Design review of the part built by this model. Coordinates are the model's own, in mm. A direction names the side the tool comes from. Coordinates: 2 decimals unless noted, no trailing zeros. Write each loop counter-clockwise with the first axis right and the second up, starting at its lowest first coordinate (ties: lowest second). Pieces come first, ordered by that corner, then holes.
Q1. Add section B-B, the plane x = 21. Give the boundary of the cut face in (y, z).
Q2. Clearance check with flat-ended pins moving along their axes: pin 1 Ø8 at (y, z) = (4.5, 15) entering from +X; pin 2 Ø3 at (x, z) = (81.5, 28) entering from +Y; pin 3 Ø2 at (x, z) = (136.5, 30) entering from -Y. State where each tip first meets the part, or that it passes through.
Q3. Add section A-A, the plane z = 20. Give the boundary of the cut face in (x, y).
Q4. Machinability: for faces 5 (the face through (110, 10, 17.5)), 6 (the face through (66, 0, 20)), 7 (the face through (80.7, 18, 20)), 8 (the face through (136, 16.4, 20)), which of the approach directions +Z, -Z, +X, -X, +Y, -Y give a long, thin tool a straight path to every point of the face, cutting with its end or side? Answer none if there is none.
Q5. Add section D-D, the plane y = 35. Give the boundary of the cut face in (x, z), plus the area to 3 significant figures.
Q6. To check wall thickness, follow probe 1 along X at (y, z) = (6, 19); probe 2 along X at (y, z) = (27, 31.5); probe 3 along X at (y, z) = (23.5, 21.5). State the ranges of each line that lie inside material, in increasing order.
Q7. The part is to be moulded in two halves that separate along Y. For faces 1 (the face through (53, 11, 0)), 2 (the face through (17.9, 23, 20)), 3 (the face through (21, 26.4, 20)), 4 (the face through (12, 40, 20)), say which applies: +Y half, -Y half, draft (parallel to the pull), parting line (faces both ways), or undercut.
Q8. Add section C-C, the plane z = 26. Give the boundary of the cut face in (x, y).
Autodesk Inventor part; units mm, degrees
ref_plane "YZ Plane" through (0, 0, 0) normal (1, 0, 0) x (0, 1, 0)
ref_plane "XZ Plane" through (0, 0, 0) normal (0, 1, 0) x (-1, 0, 0)
ref_plane "XY Plane" through (0, 0, 0) normal (0, 0, 1) x (1, 0, 0)
sketch "Boceto1" plane through (0, 0, 0) normal (0, 0, 1) x (1, 0, 0)
  line L0 (0, 0) -> (134.3, 0)
  line L1 (0, 0) -> (0, 40)
  line L2 (0, 40) -> (24.3, 40)
  line L3 (24.3, 40) -> (24.3, 26.4)
  line L4 (24.3, 26.4) -> (17.9, 26.4)
  line L5 (17.9, 26.4) -> (17.9, 19.3)
  line L6 (17.9, 19.3) -> (138.6, 19.3) construction
  line L7 (134.3, 0) -> (134.3, 16.4) construction
  line L8 (134.3, 0) -> (134.3, 16.4)
  line L9 (134.3, 16.4) -> (138.6, 16.4)
  line L10 (138.6, 16.4) -> (138.6, 19.3)
  line L11 (17.9, 19.3) -> (80.7, 19.3) construction
  line L12 (80.7, 19.3) -> (80.7, 21.1) construction
  line L13 (80.7, 21.1) -> (80.7, 15.4) construction
  line L14 (17.9, 19.3) -> (80.7, 15.4)
  line L15 (80.7, 15.4) -> (80.7, 21.1)
  line L16 (80.7, 21.1) -> (138.6, 19.3)
  dimension "d0" = 134.3
  dimension "d1" = 40
  dimension "d2" = 24.3
  dimension "d3" = 13.6
  dimension "d4" = 6.4
  dimension "d5" = 7.1
  dimension "d6" = 120.7
  dimension "d7" = 16.4
  dimension "d9" = 4.3
  dimension "d10" = 62.8
  dimension "d11" = 1.8
  dimension "d12" = 5.7
extrude "Extrusión1" add sketch "Boceto1" along normal blind 40
sketch "Boceto2" plane through (0, 0, 0) normal (0, -1, 0) x (1, 0, 0)
  line L0 (0, 0) -> (79.9, 0)
  line L1 (24.3, 0) -> (0, 0)
  line L2 (79.9, 0) -> (79.9, 20)
  line L3 (0, 0) -> (134.3, 0)
  line L4 (79.9, 0) -> (99.9, 0) construction
  line L5 (79.9, 20) -> (49.9, 20)
  line L6 (80.7, 0) -> (80.7, 40)
  line L7 (79.9, 20) -> (109.9, 20) construction
  line L8 (79.9, 20) -> (109.9, 20)
  line L9 (79.9, 20) -> (109.9, 20) construction
  line L10 (47.4, 17.5) -> (52.4, 17.5)
  line L11 (52.4, 17.5) -> (52.4, 22.5)
  line L12 (52.4, 22.5) -> (47.4, 22.5)
  line L13 (47.4, 22.5) -> (47.4, 17.5)
  line L14 (47.4, 17.5) -> (52.4, 22.5) construction
  line L15 (52.4, 17.5) -> (47.4, 22.5) construction
  line L16 (107.4, 17.5) -> (112.4, 17.5)
  line L17 (112.4, 17.5) -> (112.4, 22.5)
  line L18 (112.4, 22.5) -> (107.4, 22.5)
  line L19 (107.4, 22.5) -> (107.4, 17.5)
  line L20 (107.4, 17.5) -> (112.4, 22.5) construction
  line L21 (112.4, 17.5) -> (107.4, 22.5) construction
  dimension "d15" = 79.9
  dimension "d16" = 20
  dimension "d17" = 90
  dimension "d18" = 30
  dimension "d19" = 180
  dimension "d20" = 30
  dimension "d21" = 0
  dimension "d22" = 5
  dimension "d23" = 5
  dimension "d24" = 5
  dimension "d25" = 5
extrude "Extrusión2" cut sketch "Boceto2" against normal blind 40 contours L11 L10 L13 L12 | L19 L18 L17 L16
equation "\"d15\" = Largo_segundo_boceto"
equation "\"d22\" = Espesor_corte"
equation "\"d23\" = Espesor_corte"
equation "\"d24\" = Espesor_corte"
equation "\"d25\" = Espesor_corte"
equation "\"Correccion_rebaje\" = 5"
equation "\"Espesor_corte\" = 5"
equation "\"Espesor_detalle\" = 2.5"
equation "\"Largo_segundo_boceto\" = 79.9"
properties part number "Macho_parametrizado"
Here are the results:
1. outline: (0, 0) - (19.11, 0) - (19.11, 40) - (0, 40) - close; (26.4, 0) - (40, 0) - (40, 40) - (26.4, 40) - close
2. pin 1: stops at x = 134.3
2. pin 2: stops at y = 21.1
2. pin 3: stops at y = 16.4
3. outline: (0, 0) - (47.4, 0) - (47.4, 17.47) - (17.9, 19.3) - (17.9, 26.4) - (24.3, 26.4) - (24.3, 40) - (0, 40) - close; (52.4, 0) - (107.4, 0) - (107.4, 20.27) - (80.7, 21.1) - (80.7, 15.4) - (52.4, 17.16) - close; (112.4, 0) - (134.3, 0) - (134.3, 16.4) - (138.6, 16.4) - (138.6, 19.3) - (112.4, 20.11) - close
4. face 5: +Y, -Y
4. face 6: +Z, -Z, +X, -X, -Y
4. face 7: +Z, -Z, +Y
4. face 8: +Z, -Z, +X, -Y
5. outline: (0, 0) - (24.3, 0) - (24.3, 40) - (0, 40) - close
5. area: 972 mm2
6. probe 1: x = 0 to 47.4, 52.4 to 107.4, 112.4 to 134.3
6. probe 2: x = 0 to 24.3
6. probe 3: x = 0 to 17.9
7. face 1: draft
7. face 2: undercut
7. face 3: undercut
7. face 4: +Y half
8. outline: (0, 0) - (134.3, 0) - (134.3, 16.4) - (138.6, 16.4) - (138.6, 19.3) - (80.7, 21.1) - (80.7, 15.4) - (17.9, 19.3) - (17.9, 26.4) - (24.3, 26.4) - (24.3, 40) - (0, 40) - close
